from build123d import *

# Parameters (mm, degrees)
SKETCH1_W           = 609.6
SKETCH1_H           = 203.2
BOSS_EXTRUDE1_DEPTH = 25.4
SKETCH2_R           = 2.3815
SKETCH2_R_2         = 2.5525
CUT_EXTRUDE2_DEPTH  = 26.4
CUT_EXTRUDE3_DEPTH  = 8


with BuildPart() as part:
    # Sketch1 → Boss-Extrude1 (new body)
    with BuildSketch(Plane(origin=(0, 0, 0), x_dir=(1, 0, 0), z_dir=(0, 1, 0))):
        with Locations((304.8, 101.6)):
            Rectangle(SKETCH1_W, SKETCH1_H)
    extrude(amount=BOSS_EXTRUDE1_DEPTH)

    # Sketch2 → Cut-Extrude2 (cut, through all)
    with BuildSketch(Plane(origin=(0, 25.4, 0), x_dir=(1, 0, 0), z_dir=(0, 1, 0))):
        with Locations(Location((50.8, 101.6, 0), (0, 0, 270))):  # turned: the seam where the file's is
            Circle(SKETCH2_R)
        with Locations(Location((70.8, 101.6, 0), (0, 0, 270))):  # turned: the seam where the file's is
            Circle(SKETCH2_R)
        with Locations(Location((70.8, 121.6, 0), (0, 0, 270))):  # turned: the seam where the file's is
            Circle(SKETCH2_R_2)
        with Locations(Location((70.8, 81.6, 0), (0, 0, 270))):  # turned: the seam where the file's is
            Circle(SKETCH2_R_2)
        with BuildLine():
            Line((474.530890234, 103.9815), (564.530890234, 103.9815))
            ThreePointArc((564.530890234, 103.9815), (566.912390234, 101.6), (564.530890234, 99.2185))
            Line((564.530890234, 99.2185), (474.530890234, 99.2185))
            ThreePointArc((474.530890234, 99.2185), (472.149390234, 101.6), (474.530890234, 103.9815))
        make_face()
        with BuildLine():
            Line((484.541340045, 125.1), (564.541340045, 125.1))
            ThreePointArc((564.541340045, 125.1), (568.041340045, 121.6), (564.541340045, 118.1))
            Line((564.541340045, 118.1), (484.541340045, 118.1))
            ThreePointArc((484.541340045, 118.1), (481.041340045, 121.6), (484.541340045, 125.1))
        make_face()
        with BuildLine():
            Line((484.541340045, 85.1), (564.541340045, 85.1))
            ThreePointArc((564.541340045, 85.1), (568.041340045, 81.6), (564.541340045, 78.1))
            Line((564.541340045, 78.1), (484.541340045, 78.1))
            ThreePointArc((484.541340045, 78.1), (481.041340045, 81.6), (484.541340045, 85.1))
        make_face()
    extrude(amount=-CUT_EXTRUDE2_DEPTH, mode=Mode.SUBTRACT)

    # Sketch7 → Cut-Extrude3 (cut)
    with BuildSketch(Plane.XZ):
        with BuildLine():
            Line((484.541340045, -76.1), (564.541340045, -76.1))
            ThreePointArc((564.541340045, -76.1), (570.041340045, -81.6), (564.541340045, -87.1))
            Line((564.541340045, -87.1), (484.541340045, -87.1))
            ThreePointArc((484.541340045, -87.1), (479.041340045, -81.6), (484.541340045, -76.1))
        make_face()
        with BuildLine():
            Line((484.541340045, -116.1), (564.541340045, -116.1))
            ThreePointArc((564.541340045, -116.1), (570.041340045, -121.6), (564.541340045, -127.1))
            Line((564.541340045, -127.1), (484.541340045, -127.1))
            ThreePointArc((484.541340045, -127.1), (479.041340045, -121.6), (484.541340045, -116.1))
        make_face()
    extrude(amount=-CUT_EXTRUDE3_DEPTH, mode=Mode.SUBTRACT)


solid = part.part
Model file for the job. Use its own axes, mm. A direction names the side the tool comes from. Give positions to 0.01 mm unless a question says otherwise; leave off trailing zeros. Loops run counter-clockwise (first coordinate to the right, second up) from the corner with the lowest first, then second, coordinate; pieces in that order, holes last.
Item 1: Which spindle directions (+Z, -Z, +X, -X, +Y, -Y) get a long thin tool onto all of the face, cutting with end or side? Do faces 1 (the face through (519, 13, -103.982)), 2 (the face through (525.2, 8, -77.9)), 3 (the face through (301, 25.4, -103)). Say none if no direction does.
Check values:
face 1: +Y, -Y
face 2: -Y
face 3: +Z, -Z, +X, -X, +Y
Item 2: Drop flat-ended pins along their axis: P1, Ø2.5, axis at x = 534.5, y = 5, coming from the +Z side; P2, Ø4.5, axis at x = 70.8, z = -121.6, coming from the -Y side; P3, Ø9, axis at x = 523.5, z = -81, coming from the -Y side. Give the stop position or say it passes through.
Check values:
P1: stops at z = 0
P2: passes through
P3: stops at y = 8
Item 3: Drill centre lines: line 1 along Z through (x, y) = (527.5, 19); line 2 along X through (y, z) = (9.5, -121.6); line 3 along X through (y, z) = (14.25, -101.6). Where is each one in solid material? Low to high.
Check values:
line 1: z = -203.2 to -125.1, -118.1 to -103.98, -99.22 to -85.1, -78.1 to 0
line 2: x = 0 to 68.25, 73.35 to 481.04, 568.04 to 609.6
line 3: x = 0 to 48.42, 53.18 to 68.42, 73.18 to 472.15, 566.91 to 609.6
Item 4: Mould opens along X. For faces 4 (the face through (301, 13, 0)), 5 (the face through (609.6, 13, -100)), 6 (the face through (524, 17, -85.1)) say: +X half, -X half, draft (parallel to the pull), parting line (faces both ways), or undercut.
Check values:
face 4: draft
face 5: +X half
face 6: undercut
Item 5: Slice it at A-A (x = 546). Write the cut outline in (y, z).
Check values:
outline: (0, -203.2) - (25.4, -203.2) - (25.4, -125.1) - (8, -125.1) - (8, -127.1) - (0, -127.1) - close; (0, -116.1) - (8, -116.1) - (8, -118.1) - (25.4, -118.1) - (25.4, -103.98) - (0, -103.98) - close; (0, -99.22) - (25.4, -99.22) - (25.4, -85.1) - (8, -85.1) - (8, -87.1) - (0, -87.1) - close; (0, -76.1) - (8, -76.1) - (8, -78.1) - (25.4, -78.1) - (25.4, 0) - (0, 0) - close
